Can you work these out from the model? Positions are in its coordinate system, mm. A direction names the side the tool comes from. Coordinates: 2 decimals unless noted, no trailing zeros. Order: outer loops, then holes, each group sorted by start corner. A loop starts at its lowest first (then second) coordinate and runs counter-clockwise, first axis right, second up. Notation, with made-up numbers: (-1.75, 1) -> (18.25, 1) arc R8 cw to (18.25, 15) -> close; hole circle Ø6 at (26, 26.5). An arc over 180 degrees is marked (long way). Return JSON: item names as keys, results as strings. Group by question number.
1) Thinking about a two-plate mould opening in Y: for faces 4 (the flat face through (8, 0, 4)), 5 (the cylindrical face through (-2.348, 12.278, 5.085)), 6 (the flat face through (-8, 0, 9)), 7 (the cylindrical face through (-2.72, 1.64, 4.83)), which applies, +Y half, -Y half, draft (parallel to the pull), parting line (faces both ways), or undercut?
2) For faces 1 (the flat face through (-3, -2, 0)), 2 (the flat face through (0, -6, 8.8)), 3 (the flat face through (8, 1, 5)), which set-ups out of +Z, -Z, +X, -X, +Y, -Y let a thin tool reach every point of the face, with its end or its side?
3) If we section it at B-B, the plane z = 1: Please give me the cut outline in (x, y) (3 decimals).
4) For pin 1 (6.5 mm diameter, centred on x = -1, y = -6.5, fed in from +Z); pin 2 (4.5 mm diameter, centred on x = 9.5, z = 6, fed in from +Y); pin 3 (3 mm diameter, centred on y = -6, z = 3.5, fed in from +X), each with a flat end and sliding along its axis, tell me the tip position at first contact or that it passes through.
5) If we section it at A-A, the plane x = 0: Please give me the cut outline in (y, z) (3 decimals).
6) If I drill on probe 1 along Y at (x, z) = (0, 6.25) (3 decimals); probe 2 along Z at (x, y) = (4, -0.5); probe 3 along Y at (x, z) = (9.5, 2.75), over which ranges is the centre line in solid material (lowest first)? Write a range as from..to.
from build123d import *

# Parameters (mm, degrees)
SKETCH001_R   = 12.5
SKETCH001_R_2 = 3.175
PAD_DEPTH     = 8.8
PAD002_DEPTH  = 1
FILLET_R      = 0.5
SKETCH007_W   = 9.8
SKETCH007_H   = 1
POCKET_DEPTH  = 9.8


with BuildPart() as part:
    # Sketch001 → Pad (new body)
    with BuildSketch(Plane.XY):
        Circle(SKETCH001_R)
        Circle(SKETCH001_R_2, mode=Mode.SUBTRACT)
    extrude(amount=PAD_DEPTH)

    # Sketch003 → Pad002 (new body)
    with BuildSketch(Plane.XY.offset(8.8)):
        with BuildLine():
            Line((-12.5, 0), (-3.175, 0))
            ThreePointArc((3.175, 0), (0, 3.175), (-3.175, 0))
            Line((3.175, 0), (12.5, 0))
            ThreePointArc((12.5, 0), (0, 12.5), (-12.5, 0))
        make_face()
    extrude(amount=PAD002_DEPTH)

    # Fillet
    fillet_edges = [part.edges().sort_by_distance(p)[0] for p in [
        (-12.5, 0, 0),
    ]]
    fillet(fillet_edges, radius=FILLET_R)

    # Sketch007 → Pocket (cut)
    with BuildSketch(Plane(origin=(0, 0, 0), x_dir=(1, 0, 0), z_dir=(0, 0, -1))):
        with Locations((7.7, -0.5)):
            Rectangle(SKETCH007_W, SKETCH007_H)
    extrude(amount=-POCKET_DEPTH, mode=Mode.SUBTRACT)


solid = part.part
Result sheet:
{
 "1": {"face 4": "undercut", "face 5": "parting line", "face 6": "-Y half", "face 7": "undercut"},
 "2": {"face 1": "-Z, +X, -X, +Y, -Y", "face 2": "+Z, +X, -X, -Y", "face 3": "+Z, -Z, +X"},
 "3": {"outline": "(3.013, 1) -> (12.46, 1) arc R12.5 ccw (long way) to (12.5, 0) -> (3.175, 0) arc R3.175 cw (long way) to start"},
 "4": {"pin 1": "stops at z = 8.8", "pin 2": "stops at y = 10.18", "pin 3": "stops at x = 11.66"},
 "5": {"outline": "(-12.5, 0.5) arc R0.5 ccw to (-12, 0) -> (-3.175, 0) -> (-3.175, 8.8) -> (-12.5, 8.8) -> close; (3.175, 0) -> (12, 0) arc R0.5 ccw to (12.5, 0.5) -> (12.5, 9.8) -> (3.175, 9.8) -> close"},
 "6": {"probe 1": "y = -12.5..-3.175, 3.175..12.5", "probe 2": "z = 0..8.8", "probe 3": "y = -8.12..0, 1..8.12"}
}
